Design review of the part built by this model. Coordinates are the model's own, in mm. A direction names the side the tool comes from. Round coordinates to 2 decimals unless told otherwise and drop trailing zeros. Order: outer loops, then holes, each group sorted by start corner. A loop starts at its lowest first (then second) coordinate and runs counter-clockwise, first axis right, second up.
from build123d import *

# Parameters (mm, degrees)
BOSS_EXTRUDE1_DEPTH = 25
SKETCH2_R           = 8
CUT_EXTRUDE1_DEPTH  = 11
BOSS_EXTRUDE2_DEPTH = 10
CUT_EXTRUDE2_DEPTH  = 11
BOSS_EXTRUDE3_DEPTH = 30
CUT_EXTRUDE4_DEPTH  = 41


with BuildPart() as part:
    # Sketch1 → Boss-Extrude1 (new body, symmetric)
    with BuildSketch(Plane.XY):
        with BuildLine():
            Line((30, 0), (90, 0))
            Line((90, 0), (90, 10))
            Line((90, 10), (38.729833462, 10))
            ThreePointArc((38.729833462, 10), (0, 40), (-38.729833462, 10))
            Line((-38.729833462, 10), (-90, 10))
            Line((-90, 10), (-90, 0))
            Line((-90, 0), (-30, 0))
            ThreePointArc((-30, 0), (0, 30), (30, 0))
        make_face()
    extrude(amount=BOSS_EXTRUDE1_DEPTH, both=True)

    # Sketch2 → Cut-Extrude1 (cut, through all)
    with BuildSketch(Plane(origin=(0, 10, 0), x_dir=(1, 0, 0), z_dir=(0, 1, 0))):
        with Locations(Location((-60, 0, 0), (0, 0, 180))):  # turned: the seam where the file's is
            Circle(SKETCH2_R)
        with BuildLine():
            Line((-42.759901773, 20), (-60, 20))
            ThreePointArc((-60, 20), (-79.992623239, 0.543153766), (-61.08590686, -19.970498399))
            Line((-61.08590686, -19.970498399), (-43.845808633, -19.970498399))
            ThreePointArc((-43.845808633, -19.970498399), (-40.258710631, -21.438445011), (-38.729833462, -25))
            Line((-38.729833462, -25), (-90, -25))
            Line((-90, -25), (-90, 25))
            Line((-90, 25), (-38.729833462, 25))
            ThreePointArc((-38.729833462, 25), (-39.862779167, 21.789024658), (-42.759901773, 20))
        make_face()
    cut_extrude1 = extrude(amount=-CUT_EXTRUDE1_DEPTH, mode=Mode.SUBTRACT)

    # Mirror1: Cut-Extrude1 across plane
    add(cut_extrude1.mirror(Plane(origin=(0, 0, 0), x_dir=(0, 0, 1), z_dir=(1, 0, 0))), mode=Mode.SUBTRACT)

    # Sketch3 → Boss-Extrude2 (add)
    with BuildSketch(Plane.XY.offset(25)):
        Polygon((38.729833462, 0), (-38.729833462, 0), (-25, 100), (25, 100), align=None)
    extrude(amount=BOSS_EXTRUDE2_DEPTH)

    # Sketch5 → Cut-Extrude2 (cut, through all)
    with BuildSketch(Plane(origin=(0, 0, 25), x_dir=(-1, 0, 0), z_dir=(0, 0, -1))):
        with BuildLine():
            ThreePointArc((30, 0), (0, 30), (-30, 0))
            Line((-30, 0), (30, 0))
        make_face()
    extrude(amount=-CUT_EXTRUDE2_DEPTH, mode=Mode.SUBTRACT)

    # Sketch10 → Boss-Extrude3 (add)
    with BuildSketch(Plane(origin=(0, 0, 25), x_dir=(-1, 0, 0), z_dir=(0, 0, -1))):
        with BuildLine():
            Line((-25, 100), (25, 100))
            ThreePointArc((25, 100), (0, 75), (-25, 100))
        make_face()
    extrude(amount=BOSS_EXTRUDE3_DEPTH)

    # Sketch11 → Cut-Extrude4 (cut, through all)
    with BuildSketch(Plane(origin=(0, 0, -5), x_dir=(-1, 0, 0), z_dir=(0, 0, -1))):
        with BuildLine():
            Line((15, 100), (-15, 100))
            ThreePointArc((-15, 100), (0, 85), (15, 100))
        make_face()
    extrude(amount=-CUT_EXTRUDE4_DEPTH, mode=Mode.SUBTRACT)


solid = part.part
1) The part is to be moulded in two halves that separate along X. For faces 1 (the face through (-39.83, 5.07, -21.83)), 2 (the face through (51, 5, -20)), 3 (the face through (0, 85, 15)), say which applies: released by +X, released by -X, zero draft, split by the parting line, or undercut.
Results:
face 1: released by -X
face 2: zero draft
face 3: undercut
2) Take a section at C-C on z = 27. Give the boundary of the cut face in (x, y).
Results:
outline: (-38.73, 0) - (-30, 0) arc R30 cw to (30, 0) - (38.73, 0) - (25, 100) - (15, 100) arc R15 cw to (-15, 100) - (-25, 100) - close
3) Take a section at A-A on z = 0. Give the boundary of the cut face in (x, y), plus the area to 3 significant figures.
Results:
outline: (-80, 0) - (-68, 0) - (-68, 10) - (-80, 10) - close; (-52, 0) - (-30, 0) arc R30 cw to (30, 0) - (52, 0) - (52, 10) - (38.73, 10) arc R40 ccw to (-38.73, 10) - (-52, 10) - close; (-25, 100) arc R25 ccw to (25, 100) - (15, 100) arc R15 cw to (-15, 100) - close; (68, 0) - (80, 0) - (80, 10) - (68, 10) - close
area: 2,220 mm2
4) Clearance check with flat-ended pins moving along their axes: P1, Ø8, axis at x = 51.5, y = 4, coming from the +Z side; P2, Ø12.5, axis at x = -65.5, z = 5.5, coming from the +Y side; P3, Ø5, axis at y = 44, z = -12.5, coming from the +X side; P4, Ø6, axis at x = 15, z = 23.5, coming from the -Y side. State where each tip first meets the part, or that it passes through.
Results:
P1: stops at z = 19.97
P2: stops at y = 10
P3: passes through
P4: stops at y = 24
5) To check wall thickness, follow line 1 along Z through (x, y) = (-60, 6); line 2 along Y through (x, z) = (65.5, 14.5); line 3 along X through (y, z) = (17.5, -22). State the ranges of each line that lie inside material, in increasing order.
Results:
line 1: z = -20 to -8, 8 to 19.97
line 2: y = 0 to 10
line 3: x = -35.97 to -24.37, 24.37 to 35.97
6) For faces 4 (the face through (-54, 10, 6)), 5 (the face through (53, 5, 19.97)), 6 (the face through (-31.96, 49.3, 29.93)), 7 (the face through (79.976, 5.07, -0.975)), 8 (the face through (-51, 5, -20)), list the 3-axis set-ups (+Z, -Z, +X, -X, +Y, -Y) from which the entire face can be reached by the end or side of a thin tool; tool diameter is ignored.
Results:
face 4: +Z, -Z, -X, +Y
face 5: +Z, +X, +Y, -Y
face 6: +Z, -X, +Y
face 7: +X, +Y, -Y
face 8: -Z, -X, +Y, -Y
7) Take a section at D-D on x = 20.5. Give the boundary of the cut face in (y, z).
Results:
outline: (21.9, -25) - (34.35, -25) - (34.35, 25) - (85.69, 25) - (85.69, -5) - (100, -5) - (100, 35) - (21.9, 35) - close
8) Take a section at B-B on y = 91. Give the boundary of the cut face in (x, z), plus the area to 3 significant figures.
Results:
outline: (-26.24, 25) - (-23.32, 25) - (-23.32, -5) - (-12, -5) - (-12, 35) - (-26.24, 35) - close; (12, -5) - (23.32, -5) - (23.32, 25) - (26.24, 25) - (26.24, 35) - (12, 35) - close
area: 964 mm2
